Could you check a few things on this model? Use its own coordinates, in mm. A direction names the side the tool comes from. Round coordinates to 2 decimals unless told otherwise and drop trailing zeros. Write each loop counter-clockwise with the first axis right and the second up, starting at its lowest first coordinate (ties: lowest second). Pieces come first, ordered by that corner, then holes. Notation, with made-up numbers: M -14.5,3 L -1.5,3 A26 cw -1.5,24 Z; hole C 29.5,51 d10. An arc over 180 degrees is marked long. One line per item, written item: value. Start each with the question number.
(1) I'm going to push flat-ended pins straight in: pin 1 Ø3.5 at (y, z) = (7.5, 5) entering from +X; pin 2 Ø2 at (x, z) = (22.5, 3.5) entering from -Y; pin 3 Ø1.5 at (y, z) = (8, 5) entering from -X. Where does each tip first touch, or does it pass through?
(2) I want a section at D-D on y = -21.5. Please give me the cut outline in (x, z), and give its area (3 significant figures).
(3) I want a section at C-C on x = 13.5. Please give me the cut outline in (y, z), and give its area (3 significant figures).
(4) If I drill on L1, parallel to Z at x = 10.5, y = 3.5; L2, parallel to Y at x = 1, z = 1.5; L3, parallel to X at y = -6.5, z = 2.1, over which ranges is the centre line in solid material (lowest first)?
(5) Thinking about a two-plate mould opening in X: for faces 3 (the face through (0, 0, 6)), 4 (the face through (17.5, 10, 5)), 5 (the face through (-29.97, 1.32, 2.96)), which applies, released by +X, released by -X, zero draft, split by the parting line, or undercut?
(6) I want a section at B-B on z = 1.5. Please give me the cut outline in (x, y).
(7) Which directions (+Z, -Z, +X, -X, +Y, -Y) give clear straight access to the entire face, cutting with the end or side of a thin tool? Please do faces 1 (the face through (0, 0, 0)), 2 (the face through (10, 10, 3)).
(8) I want a section at A-A on z = 4.75. Please give me the cut outline in (x, y).
```python
from build123d import *

# Parameters (mm, degrees)
F0_R     = 30
F1_DEPTH = 6
F2_W     = 15
F2_H     = 15
F3_DEPTH = 3


with BuildPart() as f1:
    # F0 (on Top) → F1 (new body)
    with BuildSketch(Plane.XY):
        Circle(F0_R)
    extrude(amount=F1_DEPTH)

    # F2 (on face) → F3 (cut)
    with BuildSketch(Plane.XY.offset(6)):
        with Locations((10, 10)):
            Rectangle(F2_W, F2_H)
    extrude(amount=-F3_DEPTH, mode=Mode.SUBTRACT)


solid = f1.part
```
Found:
1. pin 1: stops at x = 29.44
1. pin 2: stops at y = -20.92
1. pin 3: stops at x = -29.11
2. outline: M -20.92,0 L 20.92,0 L 20.92,6 L -20.92,6 Z
2. area: 251 mm²
3. outline: M -26.79,0 L 26.79,0 L 26.79,6 L 17.5,6 L 17.5,3 L 2.5,3 L 2.5,6 L -26.79,6 Z
3. area: 276 mm²
4. L1: z = 0 to 3
4. L2: y = -29.98 to 29.98
4. L3: x = -29.29 to 29.29
5. face 3: zero draft
5. face 4: undercut
5. face 5: split by the parting line
6. outline: C 0,0 d60
7. face 1: -Z, +X, -X, +Y, -Y
7. face 2: +Z
8. outline: C 0,0 d60; hole M 2.5,2.5 L 17.5,2.5 L 17.5,17.5 L 2.5,17.5 Z
